Could you check a few things on this drawing? It's one solid part, dimensions in mm from its lowest x, y, z. A direction names the side the tool comes from. Give positions to 0.01 mm unless a question says otherwise; leave off trailing zeros. Write each loop counter-clockwise with the first axis right and the second up, starting at its lowest first coordinate (ties: lowest second). Pieces come first, ordered by that corner, then holes.
1. Suppose I cut it at B-B (x = 28). Please give me the cut outline in (y, z), and give its area (3 significant figures).
2. If I drill on probe 1 along X at (y, z) = (4.75, 9.25); probe 2 along Z at (x, y) = (49, 4); probe 3 along Z at (x, y) = (75, 1), over which ranges is the centre line in solid material (lowest first)?
3. Thinking about a two-plate mould opening in X: for the marked faces 1, 2 and 3, which applies, pulls with the +X half, pulls with the -X half, needs draft (parallel to the pull), parting line crosses it, or undercut?
4. Suppose I cut it at C-C (x = 73.5). Please give me the cut outline in (y, z).
5. I'm going to push flat-ended pins straight in: pin 1 (1.9 mm diameter, centred on x = 52.5, y = 5, fed in from -Z); pin 2 (3 mm diameter, centred on y = 3.5, z = 4.5, fed in from +X); pin 3 (0.8 mm diameter, centred on y = 3, z = 21, fed in from -X) (1 decimal). Where does each tip first touch, or does it pass through?
6. On a 3-axis mill with a long thin cutter (end or side, diameter ignored), from which of +Z, -Z, +X, -X, +Y, -Y can I reach the whole of each face in a straight line? I mean the marked faces 4 and 5. Say none if no direction works.
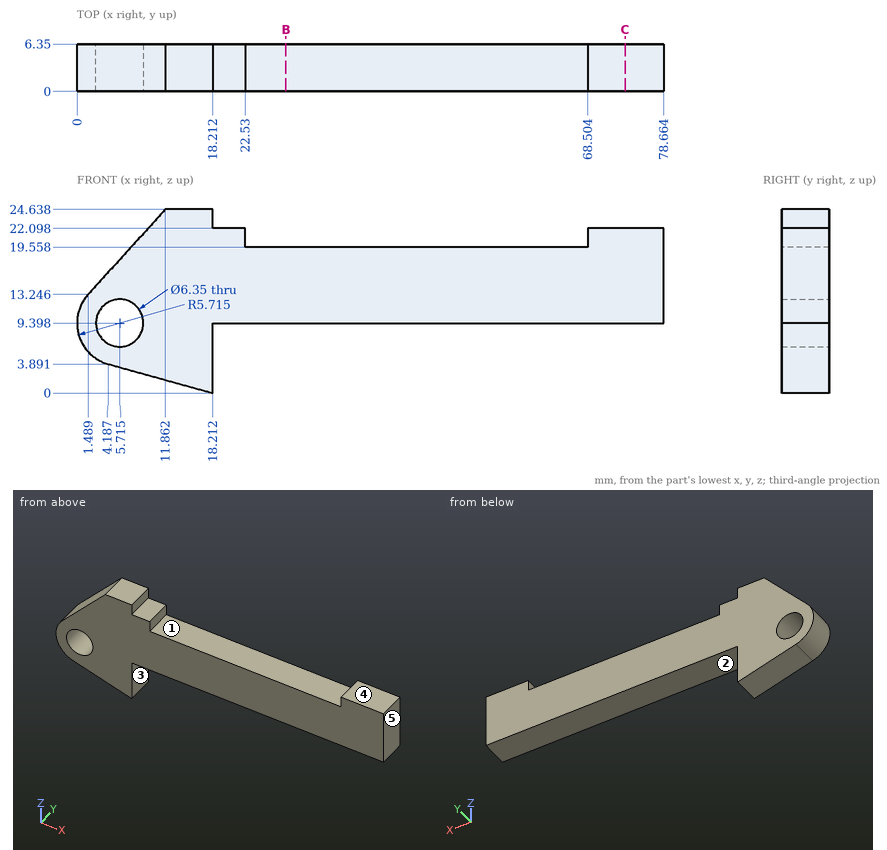
Checks:
1. outline: (0, 9.4) - (6.35, 9.4) - (6.35, 19.56) - (0, 19.56) - close
1. area: 64.5 mm2
2. probe 1: x = 0 to 2.54, 8.89 to 18.21
2. probe 2: z = 9.4 to 19.56
2. probe 3: z = 9.4 to 22.1
3. face 1: undercut
3. face 2: needs draft
3. face 3: pulls with the +X half
4. outline: (0, 9.4) - (6.35, 9.4) - (6.35, 22.1) - (0, 22.1) - close
5. pin 1: stops at z = 9.4
5. pin 2: stops at x = 18.21
5. pin 3: stops at x = 8.2
6. face 4: +Z, +X, +Y, -Y
6. face 5: +Z, -Z, +X, +Y, -Y
